from build123d import *

# Parameters (mm, degrees)
SKETCH_1_R               = 8
EXTRUDE_1_DEPTH          = 16
FILLET_1_R               = 10
CUT_EXTRUDE_1_DEPTH      = 26.455844296
CUT_EXTRUDE_1_DEPTH_BACK = 26.455844296
SKETCH_3_R               = 1.65
CUT_EXTRUDE_2_DEPTH      = 8
SKETCH_6_R               = 3.25
CUT_EXTRUDE_3_DEPTH      = 7.5
FILLET_2_R               = 1


with BuildPart() as part:
    # 草图1 → 凸台-拉伸1 (new body)
    with BuildSketch(Plane(origin=(0, 0, 0), x_dir=(1, 0, 0), z_dir=(0, 1, 0))):
        with Locations(Location((0, 0, 0), (0, 0, 270))):
            Circle(SKETCH_1_R)
        with BuildLine():
            Line((3, -4), (-3, -4))
            ThreePointArc((-3, -4), (0, 5), (3, -4))
        make_face(mode=Mode.SUBTRACT)
    extrude(amount=EXTRUDE_1_DEPTH)

    # 草图2 → 旋转1 (revolve)
    with BuildSketch(Plane.XY, mode=Mode.PRIVATE) as revolve_1_sk:
        Polygon((8, 16), (13, 16), (9, 8), (14, 0), (8, 0), align=None)
    revolve(revolve_1_sk.sketch.rotate(Axis((0, 19.267994754, 0), (0, -1, 0)), 90), axis=Axis((0, 19.267994754, 0), (0, -1, 0)))

    # 圆角1
    fillet_1_edges = [part.edges().sort_by_distance(p)[0] for p in [
        (0, 8, -9),
    ]]
    fillet(fillet_1_edges, radius=FILLET_1_R)

    # 草图3 → 切除-拉伸1 (cut, two sides: drawn at the far end of the back side and taken through both)
    with BuildSketch(Plane.XY.offset(-CUT_EXTRUDE_1_DEPTH_BACK)):
        with Locations(Location((0, 8, 0), (0, 0, 270.000000028))):
            Circle(SKETCH_3_R)
    extrude(amount=CUT_EXTRUDE_1_DEPTH + CUT_EXTRUDE_1_DEPTH_BACK, mode=Mode.SUBTRACT)

    # 草图4 → 切除-拉伸2 (cut)
    with BuildSketch(Plane.XY.offset(15)):
        Polygon((3.348631561, 8), (1.674315781, 10.9), (-1.674315781, 10.9), (-3.348631561, 8), (-1.674315781, 5.1), (1.674315781, 5.1), align=None)
    extrude(amount=-CUT_EXTRUDE_2_DEPTH, mode=Mode.SUBTRACT)

    # 草图6 → 切除-拉伸3 (cut)
    with BuildSketch(Plane.XY.offset(-15)):
        with Locations(Location((0, 8, 0), (0, 0, 180))):
            Circle(SKETCH_6_R)
    extrude(amount=CUT_EXTRUDE_3_DEPTH, mode=Mode.SUBTRACT)

    # 草图7 → 旋转2 (revolve)
    with BuildSketch(Plane.XY, mode=Mode.PRIVATE) as revolve_2_sk:
        Polygon((11.972417526, 3.244131958), (22.536438981, -4), (19, -4), (13.166853107, 0), align=None)
    revolve(revolve_2_sk.sketch.rotate(Axis((0, 21.03700922, 0), (0, -1, 0)), 90), axis=Axis((0, 21.03700922, 0), (0, -1, 0)))

    # 圆角2
    fillet_2_edges = [part.edges().sort_by_distance(p)[0] for p in [
        (0, 3.244131958, -11.97241447),
    ]]
    fillet(fillet_2_edges, radius=FILLET_2_R)

    # 草图10 → 切除-旋转1 (revolve, cut)
    with BuildSketch(Plane(origin=(0, 8, 0), x_dir=(1, 0, 0), z_dir=(0, 1, 0)), mode=Mode.PRIVATE) as cut_revolve_1_sk:
        Polygon((1.254039401, 8.908286257), (1.826463655, 10.019515519), (14.936167514, 3.266352423), (14.36374326, 2.155123161), align=None)
    revolve(cut_revolve_1_sk.sketch.rotate(Axis((14.36374326, 8, -2.155123161), (0.8889834100103146, 0, 0.45793940289784313)), 180), axis=Axis((14.36374326, 8, -2.155123161), (0.8889834100103146, 0, 0.45793940289784313)), mode=Mode.SUBTRACT)


solid = part.part
Model file for the job. Use its own axes, mm. A direction names the side the tool comes from. Give positions to 0.01 mm unless a question says otherwise; leave off trailing zeros. Order: outer loops, then holes, each group sorted by start corner. A loop starts at its lowest first (then second) coordinate and runs counter-clockwise, first axis right, second up. Notation, with made-up numbers: M 85.25,-32 L 141.25,-32 A23 cw 141.25,-7 Z; hole C 36.25,-11.5 d9. An arc over 180 degrees is marked long. Put each result on its own line as item: value. Start each with the question number.
(1) Band-saw the part on A-A on y = 1.25. Give the cut face in (x, z).
(2) Drill centre lines: L1, parallel to X at y = 8, z = -9.25; L2, parallel to Z at x = 4, y = 9.5; L3, parallel to X at y = 5.75, z = 1. Where is each one in solid material? Low to high. Write a range as [from, to].
(3) Pin check, flat tips, straight feed: pin 1 Ø3 at (x, y) = (0, 8) entering from +Z; pin 2 Ø5 at (x, y) = (-1, 11.5) entering from -Z; pin 3 Ø12 at (x, y) = (-15, 12) entering from -Z; pin 4 Ø1.5 at (x, y) = (7.5, -1.5) entering from -Z. Stop position of each tip, or through.
(4) Pull direction Y, two halves, no side cores. Call faces 1 (the face through (2.523, 9.43, 8.826)), 2 (the face through (15, -4, -12)), 3 (the face through (-3.1, 7.02, -8.97)), 4 (the face through (0, 16, -6)): released by +Y, released by -Y, zero draft, split by the parting line, or undercut.
(5) Tool access for faces 5 (the face through (0, 0, 6)), 6 (the face through (1.4, 9.3, 7)), 7 (the face through (0, 10, 4)): list every direction of +Z, -Z, +X, -X, +Y, -Y with a clear straight run to the whole face (end or side of a thin tool).
Results below:
1. outline: C 0,0 d29.76; hole M -3,4 A5 ccw long 3,4 Z
2. L1: x = [-4.9, -3.25], [3.32, 4.9]
2. L2: z = [-9.71, -3], [3, 9.71]
2. L3: x = [-10.8, -4.9], [4.9, 10.8]
3. pin 1: passes through
3. pin 2: stops at z = -11.97
3. pin 3: stops at z = -7.76
3. pin 4: stops at z = -18.56
4. face 1: undercut
4. face 2: released by -Y
4. face 3: undercut
4. face 4: released by +Y
5. face 5: -Y
5. face 6: +Z
5. face 7: +Y, -Y
